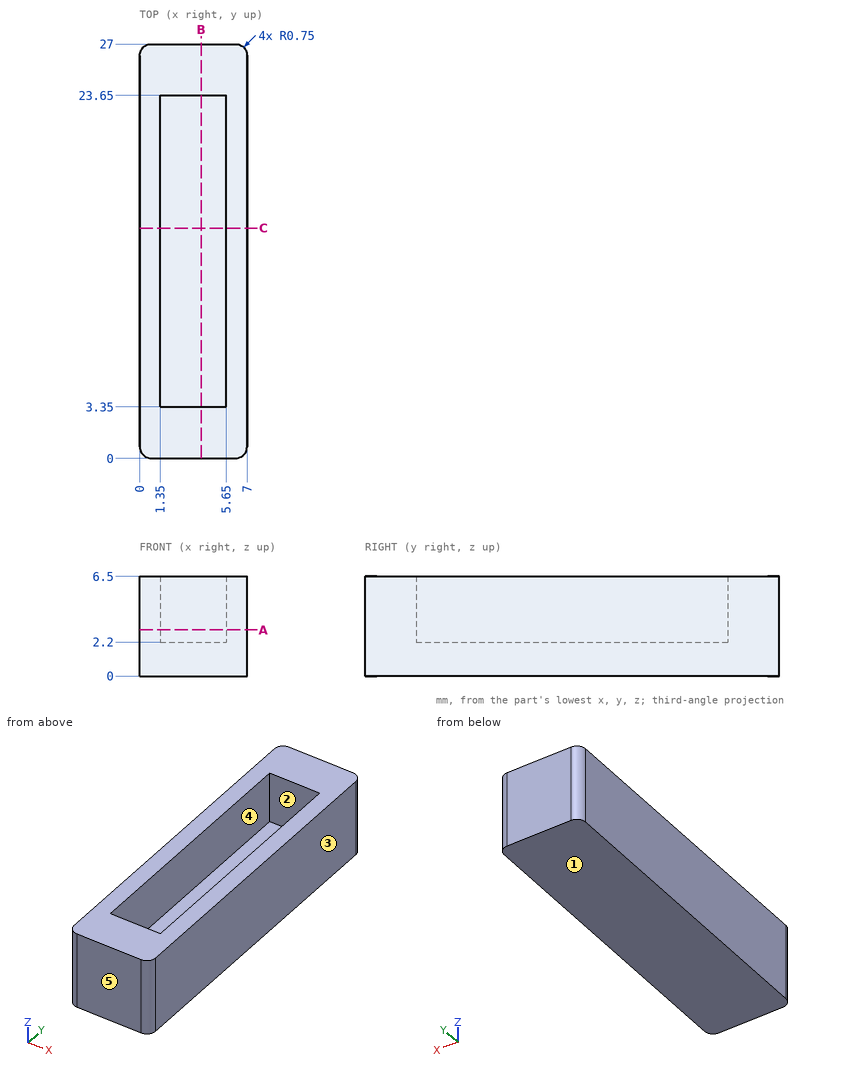
Job drawing, mm, ordinate dimensions from the low corner. One solid piece. A direction names the side the tool comes from. Round coordinates to 2 decimals unless told otherwise and drop trailing zeros. Write each loop counter-clockwise with the first axis right and the second up, starting at its lowest first coordinate (ties: lowest second). Pieces come first, ordered by that corner, then holes. Notation, with made-up numbers: (81, -27.5) -> (130, -27.5) arc R21 cw to (130, -21.5) -> close; hole circle Ø9 at (42.5, 4.25). An arc over 180 degrees is marked (long way). Answer as CSV lines item,"result".
1. Drill centre lines: line 1 (X direction, y = 11.5, z = 4.75); line 2 (Y direction, x = 3.25, z = 2.75); line 3 (Z direction, x = 3, y = 5.25). Where is each one in solid material? Low to high.
Resolved:
line 1,"0 to 1.35, 5.65 to 7"
line 2,"0 to 3.35, 23.65 to 27"
line 3,"0 to 2.2"
2. Slice it at C-C, the plane y = 15. List the corners of the cut face in (x, z), plus the area to 3 significant figures.
Resolved:
outline,"(0, 0) -> (7, 0) -> (7, 6.5) -> (5.65, 6.5) -> (5.65, 2.2) -> (1.35, 2.2) -> (1.35, 6.5) -> (0, 6.5) -> close"
area,"27.0 mm²"
3. Slice it at A-A, the plane z = 3. List the corners of the cut face in (x, y), plus the area to 3 significant figures.
Resolved:
outline,"(0, 0.75) arc R0.75 ccw to (0.75, 0) -> (6.25, 0) arc R0.75 ccw to (7, 0.75) -> (7, 26.25) arc R0.75 ccw to (6.25, 27) -> (0.75, 27) arc R0.75 ccw to (0, 26.25) -> close; hole (1.35, 3.35) -> (5.65, 3.35) -> (5.65, 23.65) -> (1.35, 23.65) -> close"
area,"101 mm²"
4. Mould opens along Y. For the marked faces 3, 4 and 5 say: +Y half, -Y half, draft (parallel to the pull), parting line (faces both ways), or undercut.
Resolved:
face 3,"draft"
face 4,"undercut"
face 5,"-Y half"
5. Slice it at B-B, the plane x = 4. List the corners of the cut face in (y, z).
Resolved:
outline,"(0, 0) -> (27, 0) -> (27, 6.5) -> (23.65, 6.5) -> (23.65, 2.2) -> (3.35, 2.2) -> (3.35, 6.5) -> (0, 6.5) -> close"
6. Pin check, flat tip, straight feed: pin 1 Ø1.3 at (x, y) = (3, 11.5) entering from +Z. Stop position of the tip, or through.
Resolved:
pin 1,"z = 2.2"
7. Tool access for the marked faces 1 and 2: list every direction of +Z, -Z, +X, -X, +Y, -Y with a clear straight run to the whole face (end or side of a thin tool).
Resolved:
face 1,"-Z, +X, -X, +Y, -Y"
face 2,"+Z"
